Read the model definition and answer for the solid it produces. Units are mm, in the model's axes. A direction names the side the tool comes from. Give positions to 0.01 mm unless a question says otherwise; leave off trailing zeros. Write each loop counter-clockwise with the first axis right and the second up, starting at its lowest first coordinate (ties: lowest second). Pieces come first, ordered by that corner, then holes. Notation, with made-up numbers: (-38.5, 78.25) -> (-18.5, 78.25) arc R21 ccw to (-18.5, 100.25) -> close; hole circle Ø6 at (-17, 2). An arc over 180 degrees is marked (long way). Write item = value, one per line.
from build123d import *

# Parameters (mm, degrees)
SKETCH_W     = 100
SKETCH_H     = 75
PAD_DEPTH    = 10
POCKET_DEPTH = 10.001


with BuildPart() as part:
    # Sketch → Pad (new body)
    with BuildSketch(Plane.XZ):
        Rectangle(SKETCH_W, SKETCH_H)
    extrude(amount=PAD_DEPTH)

    # Sketch001 → Pocket (cut, through all)
    with BuildSketch(Plane.XZ.offset(10)):
        with BuildLine():
            ThreePointArc((-35.606608, 10.606596), (-25.000001, -15), (-14.393391, 10.606594))
            Line((-18.786797, 15), (-14.393391, 10.606594))
            Line((-31.213203, 15), (-18.786797, 15))
            Line((-35.606608, 10.606596), (-31.213203, 15))
        make_face()
        with BuildLine():
            ThreePointArc((13.577536, 9.722516), (24.984095, -14.999992), (36.443057, 9.69827))
            Line((31.141327, 15), (36.443057, 9.69827))
            Line((18.85502, 15), (31.141327, 15))
            Line((13.577536, 9.722516), (18.85502, 15))
        make_face()
    extrude(amount=-POCKET_DEPTH, mode=Mode.SUBTRACT)


solid = part.part
(1) The part is cut by section A-A on x = -25. Determine the outline of the cut face in (y, z), plus the area to 3 significant figures.
Checks:
outline = (-10, -37.5) -> (0, -37.5) -> (0, -15) -> (-10, -15) -> close; (-10, 15) -> (0, 15) -> (0, 37.5) -> (-10, 37.5) -> close
area = 450 mm²
(2) For a pull along X with two mould halves and no side action, classify faces 1 (the flat face through (-1, -5, -37.5)), 2 (the flat face through (-33.441, -5.07, 12.773)), 3 (the flat face through (-50, -5, -1)) as released by +X, released by -X, zero draft, split by the parting line, or undercut.
Checks:
face_1 = zero draft
face_2 = undercut
face_3 = released by -X
(3) Consider L1, parallel to X at y = -3, z = 0; L2, parallel to Z at x = 25, y = -5.5; L3, parallel to X at y = -7, z = -3. Determine where each line is inside the solid, lowest interval first.
Checks:
L1 = -50 to -40, -10 to 10, 40 to 50
L2 = -37.5 to -15, 15 to 37.5
L3 = -50 to -39.7, -10.3 to 10.3, 39.7 to 50
(4) A tool of negligible diameter and unlimited length cuts with its end or side. For faces 4 (the flat face through (-1, -10, 1)), 5 (the flat face through (33.755, -5.07, 12.386)), from which of +Z, -Z, +X, -X, +Y, -Y can it reach the whole face along a straight path? Write none if from no direction.
Checks:
face_4 = +Z, -Z, +X, -X, -Y
face_5 = +Y, -Y
(5) The part is cut by section B-B on z = 0. Determine the outline of the cut face in (x, y), plus the area to 3 significant figures.
Checks:
outline = (-50, -10) -> (-40, -10) -> (-40, 0) -> (-50, 0) -> close; (-10, -10) -> (10, -10) -> (10, 0) -> (-10, 0) -> close; (40, -10) -> (50, -10) -> (50, 0) -> (40, 0) -> close
area = 400 mm²
(6) The part is cut by section C-C on y = -7.25. Determine the outline of the cut face in (x, z).
Checks:
outline = (-50, -37.5) -> (50, -37.5) -> (50, 37.5) -> (-50, 37.5) -> close; hole (-35.61, 10.61) arc R15 ccw (long way) to (-14.39, 10.61) -> (-18.79, 15) -> (-31.21, 15) -> close; hole (13.58, 9.72) arc R15 ccw (long way) to (36.44, 9.7) -> (31.14, 15) -> (18.86, 15) -> close
(7) Given P1, Ø12, axis at x = -24.5, z = -7, coming from the +Y side; P2, Ø2, axis at x = 12.5, z = -8.5, coming from the +Y side, each flat-ended and moving along its own axis, determine where each tip first touches the part or whether it passes through.
Checks:
P1 = through
P2 = 0
(8) The part is cut by section D-D on z = 8. Determine the outline of the cut face in (x, y).
Checks:
outline = (-50, -10) -> (-37.69, -10) -> (-37.69, 0) -> (-50, 0) -> close; (-12.31, -10) -> (12.31, -10) -> (12.31, 0) -> (-12.31, 0) -> close; (37.69, -10) -> (50, -10) -> (50, 0) -> (37.69, 0) -> close
